from build123d import *

# Parameters (mm, degrees)
SKETCH_1_W          = 20
SKETCH_1_H          = 20
SKETCH_1_W_2        = 19
SKETCH_1_H_2        = 19
EXTRUDE_1_DEPTH     = 7
SKETCH_3_W          = 20
SKETCH_3_H          = 20
EXTRUDE_2_DEPTH     = 8
SKETCH_4_R          = 6.2
EXTRUDE_3_DEPTH     = 43
SKETCH_5_R          = 4.85
CUT_EXTRUDE_1_DEPTH = 18
SKETCH_6_W          = 3
SKETCH_6_H          = 3
CUT_EXTRUDE_2_DEPTH = 10


with BuildPart() as part:
    # 草圖1 → 填料-伸長1 (new body)
    with BuildSketch(Plane(origin=(0, 0, 0), x_dir=(1, 0, 0), z_dir=(0, 1, 0))):
        with Locations((10, 10)):
            Rectangle(SKETCH_1_W, SKETCH_1_H)
        with Locations((10, 10)):
            Rectangle(SKETCH_1_W_2, SKETCH_1_H_2, mode=Mode.SUBTRACT)
    extrude(amount=EXTRUDE_1_DEPTH)

    # 草圖3 → 填料-伸長2 (add)
    with BuildSketch(Plane(origin=(0, 7, 0), x_dir=(1, 0, 0), z_dir=(0, 1, 0))):
        with Locations((10, 10)):
            Rectangle(SKETCH_3_W, SKETCH_3_H)
    extrude(amount=EXTRUDE_2_DEPTH)

    # 草圖4 → 填料-伸長3 (add)
    with BuildSketch(Plane(origin=(0, 15, 0), x_dir=(1, 0, 0), z_dir=(0, 1, 0))):
        with Locations((10, 10)):
            Circle(SKETCH_4_R)
    extrude(amount=EXTRUDE_3_DEPTH)

    # 草圖5 → 除料-伸長1 (cut)
    with BuildSketch(Plane(origin=(0, 58, 0), x_dir=(1, 0, 0), z_dir=(0, 1, 0))):
        with Locations((10, 10)):
            Circle(SKETCH_5_R)
    extrude(amount=-CUT_EXTRUDE_1_DEPTH, mode=Mode.SUBTRACT)

    # 草圖6 → 除料-伸長2 (cut)
    with BuildSketch(Plane(origin=(0, 7, 0), x_dir=(1, 0, 0), z_dir=(0, 1, 0))):
        with Locations((1.5, 18.5)):
            Rectangle(SKETCH_6_W, SKETCH_6_H)
        with Locations((18.5, 1.5)):
            Rectangle(SKETCH_6_W, SKETCH_6_H)
        with Locations((18.5, 18.5)):
            Rectangle(SKETCH_6_W, SKETCH_6_H)
        with Locations((1.5, 1.5)):
            Rectangle(SKETCH_6_W, SKETCH_6_H)
    extrude(amount=-CUT_EXTRUDE_2_DEPTH, mode=Mode.SUBTRACT)


solid = part.part
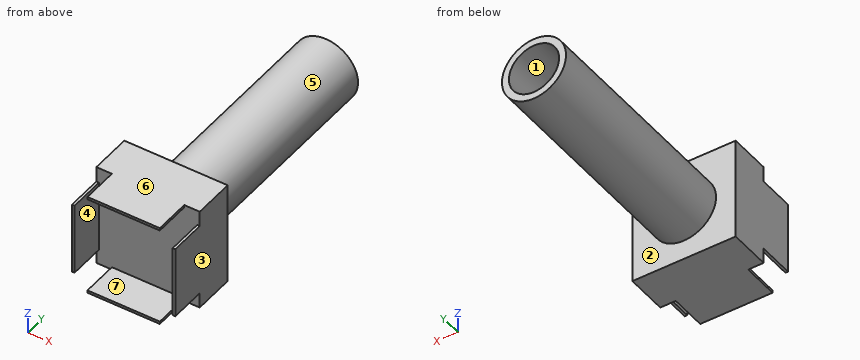
CAD build for the part. Positions are in the model's coordinates, mm. Face numbers are marked on the shaded views. A direction names the side the tool comes from. Give positions to 0.01 mm unless a question says otherwise; leave off trailing zeros. Loops run counter-clockwise (first coordinate to the right, second up) from the corner with the lowest first, then second, coordinate; pieces in that order, holes last. Notation, with made-up numbers: M 15,78 L 30,78 A17 cw 30,111 Z; hole C 59,26 d3. An arc over 180 degrees is marked long. Answer in a Markdown table with one row per item. Add a question column.
Item 1: Band-saw the part on D-D on y = 16. Give the cut face in (x, z).
Item 2: Drop flat-ended pins along their axis: P1, Ø0.6, axis at y = 4.5, z = -19.5, coming from the -X side; P2, Ø8, axis at x = 8, z = -11.5, coming from the +Y side; P3, Ø6, axis at x = 14.5, y = 51, coming from the +Z side; P4, Ø5, axis at y = 48.5, z = -12.5, coming from the -X side. Give the stop position or say it passes through.
Item 3: Band-saw the part on A-A on y = 4.5. Give the cut face in (x, z), then the cut area to 3 significant figures.
Item 4: Band-saw the part on C-C on x = 10. Give the cut face in (y, z), then the cut area to 3 significant figures.
Item 5: Band-saw the part on B-B on z = -10. Give the cut face in (x, y), then the cut area to 3 significant figures.
Item 6: Mould opens along X. For the marked faces 1, 2, 3 and 4 say: +X half, -X half, draft (parallel to the pull), parting line (faces both ways), or undercut.
Item 7: Tool access for the marked faces 5, 6 and 7: list every direction of +Z, -Z, +X, -X, +Y, -Y with a clear straight run to the whole face (end or side of a thin tool).
Item 8: Probe probe 1 along X at (y, z) = (49.5, -10); probe 2 along Z at (x, y) = (10, 52.5); probe 3 along Z at (x, y) = (3.25, 4). List the from-to ranges inside material, lowest first.
Reply:
| question | item | result |
|---|---|---|
| 1 | outline | C 10,-10 d12.4 |
| 2 | P1 | stops at x = 3 |
| 2 | P2 | stops at y = 58 |
| 2 | P3 | stops at z = -3.98 |
| 2 | P4 | stops at x = 3.8 |
| 3 | outline | M 0,-17 L 0.5,-17 L 0.5,-3 L 0,-3 Z; M 3,-20 L 17,-20 L 17,-19.5 L 3,-19.5 Z; M 3,-0.5 L 17,-0.5 L 17,0 L 3,0 Z; M 19.5,-17 L 20,-17 L 20,-3 L 19.5,-3 Z |
| 3 | area | 28.0 mm^2 |
| 4 | outline | M 0,-20 L 15,-20 L 15,-16.2 L 58,-16.2 L 58,-14.85 L 40,-14.85 L 40,-5.15 L 58,-5.15 L 58,-3.8 L 15,-3.8 L 15,0 L 0,0 L 0,-0.5 L 7,-0.5 L 7,-19.5 L 0,-19.5 Z |
| 4 | area | 526 mm^2 |
| 5 | outline | M 0,0 L 0.5,0 L 0.5,7 L 19.5,7 L 19.5,0 L 20,0 L 20,15 L 16.2,15 L 16.2,58 L 14.85,58 L 14.85,40 L 5.15,40 L 5.15,58 L 3.8,58 L 3.8,15 L 0,15 Z |
| 5 | area | 526 mm^2 |
| 6 | face 1 | undercut |
| 6 | face 2 | draft |
| 6 | face 3 | +X half |
| 6 | face 4 | undercut |
| 7 | face 5 | +Y |
| 7 | face 6 | +Z, +X, -X, +Y, -Y |
| 7 | face 7 | +X, -X, -Y |
| 8 | probe 1 | x = 3.8 to 5.15, 14.85 to 16.2 |
| 8 | probe 2 | z = -16.2 to -14.85, -5.15 to -3.8 |
| 8 | probe 3 | z = -20 to -19.5, -0.5 to 0 |
